```python
from build123d import *

# Parameters (mm, degrees)
F0_R     = 5
F0_W     = 4
F0_H     = 6
F1_DEPTH = 2
F2_R     = 5.75
F2_W     = 4
F2_H     = 6
F3_DEPTH = 1
F5_DEPTH = 10
F7_DEPTH = 8.751


with BuildPart() as f1:
    # F0 (on Top) → F1 (new body)
    with BuildSketch(Plane.XY):
        with Locations((-2, -3)):
            Circle(F0_R)
        with Locations((-2, -3)):
            Rectangle(F0_W, F0_H, mode=Mode.SUBTRACT)
    extrude(amount=F1_DEPTH)

    # F2 (on face) → F3 (join)
    with BuildSketch(Plane(origin=(0, 0, 0), x_dir=(1, 0, 0), z_dir=(0, 0, -1))):
        with Locations((-2, 3)):
            Circle(F2_R)
        with Locations((-2, 3)):
            Rectangle(F2_W, F2_H, mode=Mode.SUBTRACT)
    extrude(amount=F3_DEPTH)

    # F4 (on face) → F5 (join)
    with BuildSketch(Plane.XY.offset(2)):
        with BuildLine():
            Line((-4, -6), (-4, 0))
            Line((-4, 0), (-6, 0))
            ThreePointArc((-6, 0), (-7, -3), (-6, -6))
            Line((-6, -6), (-4, -6))
        make_face()
    extrude(amount=F5_DEPTH)

    # F6 (on face) → F7 (cut, through all)
    with BuildSketch(Plane(origin=(0, 0, 0), x_dir=(-1, 0, 0), z_dir=(0, 1, 0))):
        with BuildLine():
            Line((7, 2), (7, 11))
            ThreePointArc((7, 11), (6, 6.5), (7, 2))
        make_face()
    extrude(amount=-F7_DEPTH, mode=Mode.SUBTRACT)


solid = f1.part
```
The model under review builds one solid part; all positions refer to its coordinate system, in mm. A direction names the side the tool comes from. Give positions to 0.01 mm unless a question says otherwise; leave off trailing zeros. Write each loop counter-clockwise with the first axis right and the second up, starting at its lowest first coordinate (ties: lowest second). Pieces come first, ordered by that corner, then holes.
(1) Consider section D-D, the plane z = 4. Give the boundary of the cut face in (x, y).
(2) The part is to be moulded in two halves that separate along X. For faces 4 (the cylindrical face through (-7, -3, 1)), 5 (the flat face through (0, -3, 1)), 6 (the flat face through (0.5, -3.1, -1)), say which applies: released by +X, released by -X, zero draft, split by the parting line, or undercut.
(3) Consider section C-C, the plane z = 1.25. Give the boundary of the cut face in (x, y).
(4) Consider section A-A, the plane x = -2. Give the boundary of the cut face in (y, z), and give its area (3 significant figures).
(5) Tool access review of faces 1 (the flat face through (-5, 0, 7)), 2 (the cylindrical face through (-6.995, -3.223, 11.274)), 3 (the flat face through (-4, -3, 5)): name each direction out of +Z, -Z, +X, -X, +Y, -Y from which nothing blocks a thin tool from reaching the whole face with its end or side.
(6) For P1, Ø3, axis at y = -5.5, z = 5.5, coming from the +X side; P2, Ø2.5, axis at y = -1.5, z = 1, coming from the -X side; P3, Ø6, axis at x = 1, z = 3.5, coming from the +Y side, all flat-tipped, find the tip position at first contact; note any pin that passes through.
(7) Consider section B-B, the plane y = -3. Give the boundary of the cut face in (x, z) (3 decimals), and give its area (3 significant figures).
(8) To check wall thickness, follow L1, parallel to Y at x = -4.5, z = 9.75; L2, parallel to X at y = -4.5, z = 6.5; L3, parallel to Z at x = -1.25, y = -7.75. State the ranges of each line that lie inside material, in increasing order.
Returned:
1. outline: (-6.3, -5.55) arc R5 ccw to (-6, -6) - (-4, -6) - (-4, 0) - (-6, 0) arc R5 ccw to (-6.3, -0.45) - close
2. face 4: split by the parting line
2. face 5: undercut
2. face 6: zero draft
3. outline: circle Ø10 at (-2, -3); hole (-4, -6) - (0, -6) - (0, 0) - (-4, 0) - close
4. outline: (-8.75, -1) - (-6, -1) - (-6, 2) - (-8, 2) - (-8, 0) - (-8.75, 0) - close; (0, -1) - (2.75, -1) - (2.75, 0) - (2, 0) - (2, 2) - (0, 2) - close
4. area: 13.5 mm2
5. face 1: +Z, +X, -X, +Y
5. face 2: +Z, -X
5. face 3: +Z, -Z
6. P1: stops at x = -4
6. P2: stops at x = -7.7
6. P3: stops at y = 1.98
7. outline: (-7.75, -1) - (-4, -1) - (-4, 12) - (-7, 12) - (-7, 11) arc R10.625 cw to (-7, 2) - (-7, 0) - (-7.75, 0) - close; (0, -1) - (3.75, -1) - (3.75, 0) - (3, 0) - (3, 2) - (0, 2) - close
7. area: 43.4 mm2
8. L1: y = -6 to 0
8. L2: x = -6 to -4
8. L3: z = -1 to 2
